Geometry check sheet. Reference: the model listing, model coordinates, mm. Face numbers are marked on the shaded views. A direction names the side the tool comes from. Coordinates: 2 decimals unless noted, no trailing zeros. Loops run counter-clockwise (first coordinate to the right, second up) from the corner with the lowest first, then second, coordinate; pieces in that order, holes last.
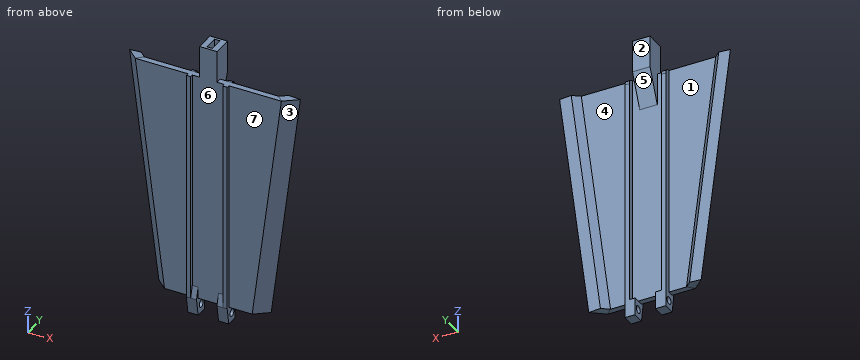
from build123d import *

# Parameters (mm, degrees)
BOSS_EXTRUDE1_DEPTH       = 2
BOSS_EXTRUDE2_DEPTH       = 6
BOSS_EXTRUDE3_DEPTH       = 6
SKETCH14_W                = 1.5
SKETCH14_H                = 79.45913029
BOSS_EXTRUDE4_DEPTH       = 2
BOSS_EXTRUDE5_DEPTH       = 11
SKETCH19_W                = 1.8
SKETCH19_H                = 4.8
CUT_EXTRUDE2_DEPTH        = 11
BOSS_EXTRUDE7_DEPTH       = 6
SKETCH21_W                = 1.5
SKETCH21_H                = 4
BOSS_EXTRUDE8_DEPTH       = 6
SKETCH24_W                = 6
SKETCH24_H                = 4
BOSS_EXTRUDE9_DEPTH       = 3.5
SKETCH25_W                = 6
SKETCH25_H                = 4
BOSS_EXTRUDE10_DEPTH      = 3.5
SKETCH22_R                = 1.25
CUT_EXTRUDE3_DEPTH        = 23.5
SKETCH27_W                = 1.5
SKETCH27_H                = 79.45913029
BOSS_EXTRUDE11_DEPTH      = 5
BOSS_EXTRUDE12_DEPTH      = 2
BOSS_EXTRUDE12_DEPTH_BACK = 1.5
BOSS_EXTRUDE13_DEPTH      = 3.5
BOSS_EXTRUDE14_DEPTH      = 2
BOSS_EXTRUDE15_DEPTH      = 2
FILLET2_R                 = 2


with BuildPart() as part:
    # Sketch1 → Boss-Extrude1 (new body)
    with BuildSketch(Plane(origin=(0, 0, 0), x_dir=(1, 0, 0), z_dir=(0, 1, 0))):
        Polygon((-21.058581006, -39.654130901), (28.941418994, -39.654130901), (18.941418994, 39.804999389), (-11.058581006, 39.804999389), align=None)
    extrude(amount=BOSS_EXTRUDE1_DEPTH)

    # Sketch2 → Cut-Loft1 section 0
    with BuildSketch(Plane.XY.offset(39.654130901)):
        Polygon((-21.058581006, 2), (-21.058581006, 0), (-19.058581006, 2), align=None)
    # Sketch3 → Cut-Loft1 section 1
    with BuildSketch(Plane(origin=(0, 0, -39.804999389), x_dir=(-1, 0, 0), z_dir=(0, 0, -1))):
        Polygon((11.058581006, 0), (11.058581006, 2), (9.058581006, 2), align=None)
    loft(mode=Mode.SUBTRACT)

    # Sketch5 → Cut-Loft2 section 0
    with BuildSketch(Plane(origin=(0, 0, -39.804999389), x_dir=(-1, 0, 0), z_dir=(0, 0, -1))):
        Polygon((-18.941418994, 0), (-18.941418994, 2), (-16.941418994, 2), align=None)
    # Sketch4 → Cut-Loft2 section 1
    with BuildSketch(Plane.XY.offset(39.654130901)):
        Polygon((28.941418994, 0), (28.941418994, 2), (26.941418994, 2), align=None)
    loft(mode=Mode.SUBTRACT)

    # Sketch6 → Boss-Extrude2 (add)
    with BuildSketch(Plane(origin=(11.881365089, 11.881365089, -1.495280032), x_dir=(-0.062677741, -0.062677741, -0.996063754), z_dir=(0.704323435, 0.704323435, -0.088639711))):
        Polygon((-41.312025236, -20.464673628), (38.461111762, -13.393605816), (38.461111762, -10.565178691), (-41.312025236, -17.636246503), align=None)
    extrude(amount=BOSS_EXTRUDE2_DEPTH)

    # Sketch7 → Boss-Extrude3 (add)
    with BuildSketch(Plane(origin=(-7.970913818, 7.970913818, -1.003146371), x_dir=(-0.062677741, 0.062677741, 0.996063754), z_dir=(-0.704323435, 0.704323435, -0.088639711))):
        Polygon((-38.955190238, -4.991170495), (40.81794676, -12.062238307), (40.81794676, -14.890665432), (-38.955190238, -7.81959762), align=None)
    extrude(amount=BOSS_EXTRUDE3_DEPTH)

    # Sketch9 → Cut-Loft3 section 0
    with BuildSketch(Plane(origin=(2.441623315, -2.441623315, -38.801853018), x_dir=(-0.998033817, -0.003936239, -0.062554018), z_dir=(0.062677741, -0.062677741, -0.996063754))):
        Polygon((17.761066429, 6.750801427), (13.768931159, 6.750801427), (15.757126317, 8.746853538), align=None)
    # Sketch8 → Cut-Loft3 section 1
    with BuildSketch(Plane(origin=(-2.558376685, 2.558376685, 40.657277272), x_dir=(0.998033817, 0.003936239, 0.062554018), z_dir=(-0.062677741, 0.062677741, 0.996063754))):
        Polygon((-22.770916709, 1.760671151), (-18.778781439, 1.760671151), (-20.766976597, 3.756723262), align=None)
    loft(mode=Mode.SUBTRACT)

    # Sketch13 → Cut-Loft4 section 0
    with BuildSketch(Plane(origin=(2.589344408, 2.589344408, 41.149410933), x_dir=(0.998033817, -0.003936239, -0.062554018), z_dir=(0.062677741, 0.062677741, 0.996063754))):
        Polygon((30.638255597, 1.760671151), (26.646120328, 1.760671151), (28.634315485, 3.756723262), align=None)
    # Sketch12 → Cut-Loft4 section 1
    with BuildSketch(Plane(origin=(-2.410655592, -2.410655592, -38.309719357), x_dir=(-0.998033817, 0.003936239, 0.062554018), z_dir=(-0.062677741, -0.062677741, -0.996063754))):
        Polygon((-25.628405317, 6.750801427), (-21.636270047, 6.750801427), (-23.624465205, 8.746853538), align=None)
    loft(mode=Mode.SUBTRACT)

    # Sketch14 → Boss-Extrude4 (add)
    with BuildSketch(Plane(origin=(0, 2, 0), x_dir=(1, 0, 0), z_dir=(0, 1, 0))):
        with Locations((10.191418994, 0.075434244)):
            Rectangle(SKETCH14_W, SKETCH14_H)
        with Locations((-2.308581006, 0.075434244)):
            Rectangle(SKETCH14_W, SKETCH14_H)
    extrude(amount=BOSS_EXTRUDE4_DEPTH)

    # Sketch15 → Boss-Extrude5 (add)
    with BuildSketch(Plane.XY.offset(39.654130901)):
        Polygon((3.941418994, 0), (6.941418994, 0), (6.941418994, 6.6), (0.941418994, 6.6), (0.941418994, 0), align=None)
    extrude(amount=BOSS_EXTRUDE5_DEPTH)

    # Sketch19 → Cut-Extrude2 (cut)
    with BuildSketch(Plane.XY.offset(50.654130901)):
        with Locations((3.941418994, 3.3)):
            Rectangle(SKETCH19_W, SKETCH19_H)
    extrude(amount=-CUT_EXTRUDE2_DEPTH, mode=Mode.SUBTRACT)

    # Sketch20 → Boss-Extrude7 (add)
    with BuildSketch(Plane.ZY.offset(-0.941418994)):
        Polygon((39.654130901, 2), (28.654130901, 2), (39.654130901, 6.6), align=None)
    extrude(amount=-BOSS_EXTRUDE7_DEPTH)

    # Sketch21 → Boss-Extrude8 (add)
    with BuildSketch(Plane(origin=(0, 0, -39.804999389), x_dir=(-1, 0, 0), z_dir=(0, 0, -1))):
        with Locations((-10.191418994, 2)):
            Rectangle(SKETCH21_W, SKETCH21_H)
        with Locations((2.308581006, 2)):
            Rectangle(SKETCH21_W, SKETCH21_H)
    extrude(amount=BOSS_EXTRUDE8_DEPTH)

    # Sketch24 → Boss-Extrude9 (add)
    with BuildSketch(Plane.ZY.offset(3.058581006)):
        with Locations((-42.804999389, 2)):
            Rectangle(SKETCH24_W, SKETCH24_H)
    extrude(amount=-BOSS_EXTRUDE9_DEPTH)

    # Sketch25 → Boss-Extrude10 (add)
    with BuildSketch(Plane(origin=(10.941418994, 0, 0), x_dir=(0, 0, -1), z_dir=(1, 0, 0))):
        with Locations((42.804999389, 2)):
            Rectangle(SKETCH25_W, SKETCH25_H)
    extrude(amount=-BOSS_EXTRUDE10_DEPTH)

    # Sketch22 → Cut-Extrude3 (cut)
    with BuildSketch(Plane(origin=(10.941418994, 0, 0), x_dir=(0, 0, -1), z_dir=(1, 0, 0))):
        with Locations((42.804999389, 2)):
            Circle(SKETCH22_R)
    extrude(amount=-CUT_EXTRUDE3_DEPTH, mode=Mode.SUBTRACT)

    # Sketch27 → Boss-Extrude11 (add)
    with BuildSketch(Plane(origin=(0, 4, 0), x_dir=(1, 0, 0), z_dir=(0, 1, 0))):
        with Locations((-2.308581006, 0.075434244)):
            Rectangle(SKETCH27_W, SKETCH27_H)
        with Locations((10.191418994, 0.075434244)):
            Rectangle(SKETCH27_W, SKETCH27_H)
    extrude(amount=-BOSS_EXTRUDE11_DEPTH)

    # Sketch28 → Boss-Extrude12 (add, two sides)
    with BuildSketch(Plane(origin=(-1.558581006, 0, 0), x_dir=(0, 0, -1), z_dir=(1, 0, 0))) as boss_extrude12_sk:
        Polygon((39.804999389, -1), (39.804999389, 0), (45.848869538, 0), align=None)
    extrude(amount=BOSS_EXTRUDE12_DEPTH)
    extrude(boss_extrude12_sk.sketch, amount=-BOSS_EXTRUDE12_DEPTH_BACK)

    # Sketch29 → Boss-Extrude13 (add)
    with BuildSketch(Plane(origin=(10.941418994, 0, 0), x_dir=(0, 0, -1), z_dir=(1, 0, 0))):
        Polygon((39.804999389, 0), (45.804999389, 0), (39.804999389, -1), align=None)
    extrude(amount=-BOSS_EXTRUDE13_DEPTH)

    # Sketch31 → Boss-Extrude14 (add)
    with BuildSketch(Plane(origin=(-1.558581006, 0, 0), x_dir=(0, 0, -1), z_dir=(1, 0, 0))):
        Polygon((39.804999389, -1), (35.804999389, 0), (39.804999389, 0), align=None)
    extrude(amount=BOSS_EXTRUDE14_DEPTH)

    # Sketch32 → Boss-Extrude15 (add)
    with BuildSketch(Plane.ZY.offset(-9.441418994)):
        Polygon((-39.804999389, 0), (-39.804999389, -1), (-35.804999389, 0), align=None)
    extrude(amount=BOSS_EXTRUDE15_DEPTH)

    # Fillet2
    fillet2_edges = [part.edges().sort_by_distance(p)[0] for p in [
        (10.191418994, 4, 39.654130901),
        (-2.308581006, 4, 39.654130901),
    ]]
    fillet(fillet2_edges, radius=FILLET2_R)


solid = part.part
(1) Scan lines: L1, parallel to X at y = 2.5, z = 44.5; L2, parallel to X at y = -0.5, z = -33.5; L3, parallel to X at y = 2.25, z = 24. Record each from-to range of solid material in increasing order.
Findings:
L1: x = 0.94 to 3.04, 4.84 to 6.94
L2: x = -3.06 to -1.56, 9.44 to 10.94
L3: x = -21.37 to -17.34, -3.06 to -1.56, 9.44 to 10.94, 25.23 to 29.26
(2) Draft check along X on the marked faces 1, 2 and 3. Enter one of: +X half, -X half, draft (parallel to the pull), parting line (faces both ways), or undercut.
Findings:
face 1: undercut
face 2: draft
face 3: +X half
(3) Access from +Z, -Z, +X, -X, +Y, -Y to the whole of each face (thin tool, end or side, straight path). Record for the marked faces 4, 5, 6 and 7.
Findings:
face 4: +Z, +Y
face 5: -Z, +Y
face 6: +Z, -Y
face 7: +Z, -Z, +X, -Y
(4) Sectioned sample at A-A on x = -7. Record the cut outline in (y, z) (3 decimals), and give its area (3 significant figures).
Findings:
outline: (0, -39.805) - (2, -39.805) - (2, 39.654) - (0, 39.654) - close
area: 159 mm2
(5) Gauge pin test, flat ends, axial feed: pin 1 Ø1.4 at (x, z) = (4, 46.5) entering from -Y; pin 2 Ø2 at (y, z) = (2.5, -15.5) entering from -X; pin 3 Ø1.6 at (x, y) = (-6, 1.5) entering from -Z (3 decimals). Record the tip position at first contact, or that the pin passes through.
Findings:
pin 1: stops at y = 0
pin 2: stops at x = -17.68
pin 3: stops at z = -39.805
